The model under review builds one solid part; all positions refer to its coordinate system, in mm. Face numbers are marked on the shaded views. A direction names the side the tool comes from. Coordinates: 2 decimals unless noted, no trailing zeros. Write each loop counter-clockwise with the first axis right and the second up, starting at its lowest first coordinate (ties: lowest second). Pieces come first, ordered by that corner, then holes.
```python
from build123d import *

# Parameters (mm, degrees)
F0_W     = 63
F0_H     = 18
F1_DEPTH = 93
F2_T     = -2
F4_DEPTH = 93
F6_DEPTH = 63
F7_R     = 1.19999


# Not quite as in the source:
# - a fillet or chamfer is up to 0.001 mm smaller than in the source, because OpenCascade refuses the exact size


with BuildPart() as f1:
    # F0 (on Front) → F1 (new body)
    with BuildSketch(Plane.XZ):
        with Locations((31.5, -9)):
            Rectangle(F0_W, F0_H)
    extrude(amount=-F1_DEPTH)

    # F2
    f2_openings = [f1.faces().sort_by_distance(p)[0] for p in [
        (31.5, 46.5, 0),
    ]]
    offset(amount=F2_T, openings=f2_openings)

    # F3 (on face) → F4 (join, through all)
    with BuildSketch(Plane.XZ):
        Polygon((0, 2), (0, 0), (1.2, 0), (2, 1), (2, 2), align=None)
        Polygon((61, 1), (61.8, 0), (63, 0), (63, 2), (61, 2), align=None)
    extrude(amount=-F4_DEPTH)

    # F5 (on face) → F6 (join, through all)
    with BuildSketch(Plane.YZ.offset(63)):
        Polygon((93, 0), (93, 2), (91, 2), (91, 1), (91.8, 0), align=None)
    extrude(amount=-F6_DEPTH)

    # F7 (radius 1.2 in the source; OpenCascade refuses exactly that, so slightly less here)
    f7_edges = [f1.edges().sort_by_distance(p)[0] for p in [
        (63, 0, -8),
        (63, 93, -8),
        (0, 0, -8),
        (0, 93, -8),
    ]]
    fillet(f7_edges, radius=F7_R)


solid = f1.part
```
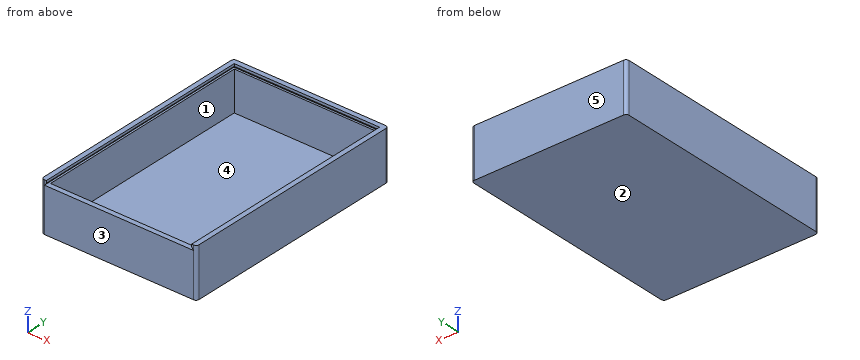
Item 1: Machinability: for the marked faces 1 and 2, which of the approach directions +Z, -Z, +X, -X, +Y, -Y give a long, thin tool a straight path to every point of the face, cutting with its end or side? Answer none if there is none.
Solved:
face 1: +Z
face 2: -Z, +X, -X, +Y, -Y
Item 2: Take a section at C-C, the plane x = 33.5. Write out the cut boundary in (y, z), plus the area to 3 significant figures.
Solved:
outline: (0, -18) - (93, -18) - (93, 2) - (91, 2) - (91, 1) - (91.8, 0) - (91, 0) - (91, -16) - (2, -16) - (2, 0) - (0, 0) - close
area: 254 mm2
Item 3: Take a section at B-B, the plane z = -9.5. Write out the cut boundary in (x, y), plus the area to 3 significant figures.
Solved:
outline: (0, 1.2) arc R1.2 ccw to (1.2, 0) - (61.8, 0) arc R1.2 ccw to (63, 1.2) - (63, 91.8) arc R1.2 ccw to (61.8, 93) - (1.2, 93) arc R1.2 ccw to (0, 91.8) - close; hole (2, 2) - (61, 2) - (61, 91) - (2, 91) - close
area: 607 mm2
Item 4: For pin 1 (18 mm diameter, centred on x = 46, y = 48.5, fed in from +Z); pin 2 (0.8 mm diameter, centred on x = 28.5, z = 1.5, fed in from -Y), all flat-tipped, find the tip position at first contact; note any pin that passes through.
Solved:
pin 1: stops at z = -16
pin 2: stops at y = 91
Item 5: Mouldability with a two-part tool opening along Y and no side actions: class the marked faces 3, 4 and 5 as pulls with the +Y half, pulls with the -Y half, needs draft (parallel to the pull), parting line crosses it, or undercut.
Solved:
face 3: pulls with the -Y half
face 4: undercut
face 5: pulls with the +Y half
Item 6: Take a section at A-A, the plane y = 22. Write out the cut boundary in (x, z), plus the area to 3 significant figures.
Solved:
outline: (0, -18) - (63, -18) - (63, 2) - (61, 2) - (61, 1) - (61.8, 0) - (61, 0) - (61, -16) - (2, -16) - (2, 0) - (1.2, 0) - (2, 1) - (2, 2) - (0, 2) - close
area: 197 mm2
Item 7: To check wall thickness, follow line 1 along X through (y, z) = (67, -4); line 2 along Y through (x, z) = (21.5, -4.25); line 3 along Z through (x, y) = (17.5, 86). State the ranges of each line that lie inside material, in increasing order.
Solved:
line 1: x = 0 to 2, 61 to 63
line 2: y = 0 to 2, 91 to 93
line 3: z = -18 to -16
